```python
from build123d import *

# Parameters (mm, degrees)
BOSS_EXTRU_1_DEPTH           = 3
R_P_TITION_CIRCULAIRE2_COUNT = 7
ESQUISSE5_R                  = 4.5
BOSS_EXTRU_2_DEPTH           = 3


with BuildPart() as part:
    # Esquisse4 → Boss.-Extru.1 (new body)
    with BuildSketch(Plane.XY):
        with BuildLine():
            Line((0, 6.577848346), (0, 4.5))
            ThreePointArc((0, 4.5), (1.039097311, 4.378387463), (2.022031395, 4.020123013))
            Line((2.022031395, 4.020123013), (2.955692415, 5.876391002))
            ThreePointArc((2.955692415, 5.876391002), (3.02541978, 7.297456647), (2.538901994, 8.634464469))
            ThreePointArc((2.538901994, 8.634464469), (2.078194622, 8.756774927), (1.611657757, 8.854521968))
            ThreePointArc((1.611657757, 8.854521968), (0.576250392, 7.878703818), (0, 6.577848346))
        make_face()
    extrude(amount=BOSS_EXTRU_1_DEPTH)


with BuildPart() as r_p_tition_circulaire2_1:
    # R_p_tition circulaire2: pattern copy
    add(part.part.rotate(Axis((0, 0, 0), (0, 0, 1)), 1 * 360 / R_P_TITION_CIRCULAIRE2_COUNT))


with BuildPart() as r_p_tition_circulaire2_2:
    # R_p_tition circulaire2: pattern copy
    add(part.part.rotate(Axis((0, 0, 0), (0, 0, 1)), 2 * 360 / R_P_TITION_CIRCULAIRE2_COUNT))


with BuildPart() as r_p_tition_circulaire2_3:
    # R_p_tition circulaire2: pattern copy
    add(part.part.rotate(Axis((0, 0, 0), (0, 0, 1)), 3 * 360 / R_P_TITION_CIRCULAIRE2_COUNT))


with BuildPart() as r_p_tition_circulaire2_4:
    # R_p_tition circulaire2: pattern copy
    add(part.part.rotate(Axis((0, 0, 0), (0, 0, 1)), 4 * 360 / R_P_TITION_CIRCULAIRE2_COUNT))


with BuildPart() as r_p_tition_circulaire2_5:
    # R_p_tition circulaire2: pattern copy
    add(part.part.rotate(Axis((0, 0, 0), (0, 0, 1)), 5 * 360 / R_P_TITION_CIRCULAIRE2_COUNT))


with BuildPart() as r_p_tition_circulaire2_6:
    # R_p_tition circulaire2: pattern copy
    add(part.part.rotate(Axis((0, 0, 0), (0, 0, 1)), 6 * 360 / R_P_TITION_CIRCULAIRE2_COUNT))


with BuildPart() as part_1:
    add(part.part)

    add(r_p_tition_circulaire2_1.part)  # Boss.-Extru.2 merges R_p_tition circulaire2_1

    add(r_p_tition_circulaire2_2.part)  # Boss.-Extru.2 merges R_p_tition circulaire2_2

    add(r_p_tition_circulaire2_3.part)  # Boss.-Extru.2 merges R_p_tition circulaire2_3

    add(r_p_tition_circulaire2_4.part)  # Boss.-Extru.2 merges R_p_tition circulaire2_4

    add(r_p_tition_circulaire2_5.part)  # Boss.-Extru.2 merges R_p_tition circulaire2_5

    add(r_p_tition_circulaire2_6.part)  # Boss.-Extru.2 merges R_p_tition circulaire2_6
    # Esquisse5 → Boss.-Extru.2 (add)
    with BuildSketch(Plane.XY):
        Circle(ESQUISSE5_R)
    extrude(amount=BOSS_EXTRU_2_DEPTH)


solid = part_1.part
```
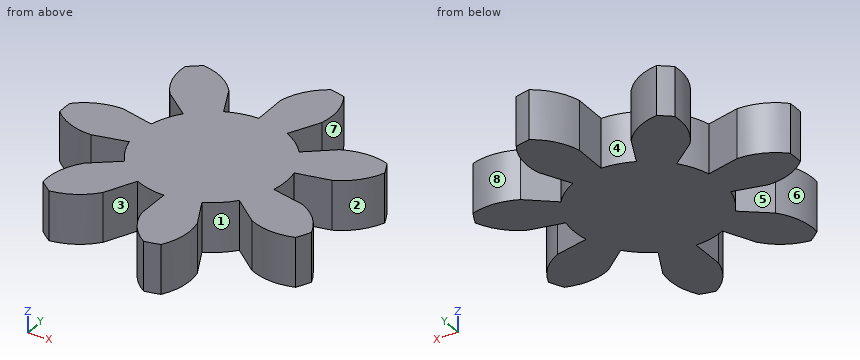
The model under review builds one solid part; all positions refer to its coordinate system, in mm. Face numbers are marked on the shaded views. A direction names the side the tool comes from. Give positions to 0.01 mm unless a question says otherwise; leave off trailing zeros. Write each loop counter-clockwise with the first axis right and the second up, starting at its lowest first coordinate (ties: lowest second). Pieces come first, ordered by that corner, then holes. Notation, with made-up numbers: M 56.5,8 L 111.5,8 A30 cw 111.5,38 Z; hole C 40,76 d10. An arc over 180 degrees is marked long. Write item = value, one per line. Start each with the question number.
Q1. Clearance check with a flat-ended pin moving along its axis: pin 1 (1 mm diameter, centred on y = 5, z = 1.5, fed in from -X). State where the tip first meets the part, or that it passes through.
Q2. Machinability: for the marked faces 1, 2, 3, 4 and 5, which of the approach directions +Z, -Z, +X, -X, +Y, -Y give a long, thin tool a straight path to every point of the face, cutting with its end or side? Answer none if there is none.
Q3. For line 1 (Y direction, x = 2.5, z = 0.95); line 2 (Y direction, x = -1, z = 1.65); line 3 (Y direction, x = 2.25, z = 0.7), list the stretches that pass through material, from the lowest coordinate up.
Q4. We need section B-B (y = -2.5). State the section outline as (x, z) points.
Q5. We need section A-A (y = 6.25). State the section outline as (x, z) points, plus the area to 3 significant figures.
Q6. We need section C-C (x = -2.25). State the section outline as (y, z) points, plus the area to 3 significant figures.
Q7. Mouldability with a two-part tool opening along X and no side actions: class the marked faces 6, 7 and 8 as released by +X, released by -X, zero draft, split by the parting line, or undercut.
Result set:
q1.pin_1 = -5.84
q2.face_1 = +Z, -Z
q2.face_2 = +Z, -Z, +X
q2.face_3 = +Z, -Z, -Y
q2.face_4 = +Z, -Z, +Y
q2.face_5 = +Z, -Z, -X
q3.line_1 = -8.49 to -5.19, -3.74 to 3.74, 4.97 to 8.65
q3.line_2 = -4.39 to 4.39
q3.line_3 = -8.71 to -4.67, -3.9 to 3.9, 4.47 to 8.71
q4.outline = M -3.74,0 L 7.71,0 L 7.71,3 L -3.74,3 Z
q5.outline = M -5.94,0 L -2.98,0 L -2.98,3 L -5.94,3 Z; M 0,0 L 3.03,0 L 3.03,3 L 0,3 Z
q5.area = 18.0 mm2
q6.outline = M -4.67,0 L 4.89,0 L 4.89,3 L -4.67,3 Z
q6.area = 28.7 mm2
q7.face_6 = released by -X
q7.face_7 = released by +X
q7.face_8 = undercut
